For this review, take the finished solid that the model builds, in its own axes (mm). Face numbers are marked on the shaded views. A direction names the side the tool comes from. Give positions to 0.01 mm unless a question says otherwise; leave off trailing zeros. Loops run counter-clockwise (first coordinate to the right, second up) from the corner with the lowest first, then second, coordinate; pieces in that order, holes last. Notation, with made-up numbers: (-24, 78) - (1, 78) arc R8 cw to (1, 91) - close; hole circle Ø8 at (27.5, 17). An arc over 180 degrees is marked (long way). Put each result on its own line as item: value.
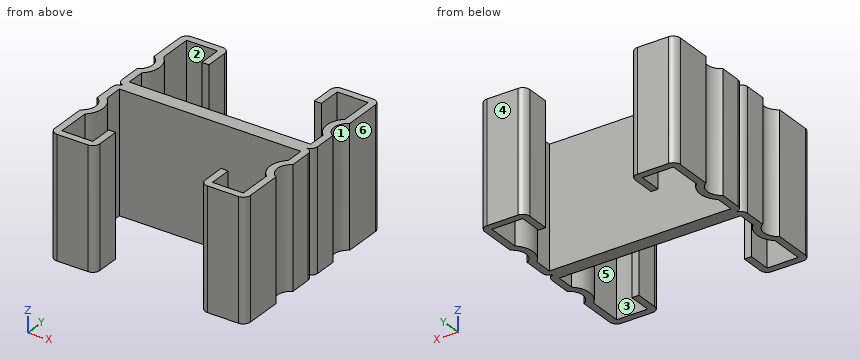
from build123d import *

# Parameters (mm, degrees)
BASE_EXTRUDE_DEPTH = 12.7


with BuildPart() as part:
    # Sketch1 → Base-Extrude (new, symmetric)
    with BuildSketch(Plane.XY):
        with BuildLine():
            Line((-20.6375, 19.1389), (-20.6375, 11.29515134))
            ThreePointArc((-20.6375, 11.29515134), (-19.1389, 8.6995), (-20.6375, 6.10384866))
            Line((-20.6375, 6.10384866), (-20.6375, 1.4986))
            ThreePointArc((-20.6375, 1.4986), (-20.198570222, 0.438929778), (-19.1389, 0))
            Line((-19.1389, 0), (19.1389, 0))
            ThreePointArc((19.1389, 0), (20.198570222, 0.438929778), (20.6375, 1.4986))
            Line((20.6375, 1.4986), (20.6375, 6.10384866))
            ThreePointArc((20.6375, 6.10384866), (19.1389, 8.6995), (20.6375, 11.29515134))
            Line((20.6375, 11.29515134), (20.6375, 19.1389))
            ThreePointArc((20.6375, 19.1389), (20.198570222, 20.198570222), (19.1389, 20.6375))
            Line((19.1389, 20.6375), (12.6111, 20.6375))
            ThreePointArc((12.6111, 20.6375), (11.551429778, 20.198570222), (11.1125, 19.1389))
            Line((11.1125, 19.1389), (11.1125, 14.2875))
            Line((11.1125, 14.2875), (12.6111, 14.2875))
            Line((12.6111, 14.2875), (12.6111, 19.1389))
            Line((12.6111, 19.1389), (19.1389, 19.1389))
            Line((19.1389, 19.1389), (19.1389, 12.050471471))
            ThreePointArc((19.1389, 12.050471471), (17.6403, 8.6995), (19.1389, 5.348528529))
            Line((19.1389, 5.348528529), (19.1389, 1.4986))
            Line((19.1389, 1.4986), (-19.1389, 1.4986))
            Line((-19.1389, 1.4986), (-19.1389, 5.348528529))
            ThreePointArc((-19.1389, 5.348528529), (-17.6403, 8.6995), (-19.1389, 12.050471471))
            Line((-19.1389, 12.050471471), (-19.1389, 19.1389))
            Line((-19.1389, 19.1389), (-12.6111, 19.1389))
            Line((-12.6111, 19.1389), (-12.6111, 14.2875))
            Line((-12.6111, 14.2875), (-11.1125, 14.2875))
            Line((-11.1125, 14.2875), (-11.1125, 19.1389))
            ThreePointArc((-11.1125, 19.1389), (-11.551429778, 20.198570222), (-12.6111, 20.6375))
            Line((-12.6111, 20.6375), (-19.1389, 20.6375))
            ThreePointArc((-19.1389, 20.6375), (-20.198570222, 20.198570222), (-20.6375, 19.1389))
        make_face()
    base_extrude = extrude(amount=BASE_EXTRUDE_DEPTH, both=True)

    # Mirror1: Base-Extrude across plane
    add(base_extrude.mirror(Plane.ZX))


solid = part.part
1) Take a section at A-A on y = 15. State the section outline as (x, z) points, and give its area (3 significant figures).
Geometry check:
outline: (-20.64, -12.7) - (-19.14, -12.7) - (-19.14, 12.7) - (-20.64, 12.7) - close; (-12.61, -12.7) - (-11.11, -12.7) - (-11.11, 12.7) - (-12.61, 12.7) - close; (11.11, -12.7) - (12.61, -12.7) - (12.61, 12.7) - (11.11, 12.7) - close; (19.14, -12.7) - (20.64, -12.7) - (20.64, 12.7) - (19.14, 12.7) - close
area: 152 mm²
2) Take a section at B-B on y = 2.5. State the section outline as (x, z) points.
Geometry check:
outline: (-20.64, -12.7) - (-19.14, -12.7) - (-19.14, 12.7) - (-20.64, 12.7) - close; (19.14, -12.7) - (20.64, -12.7) - (20.64, 12.7) - (19.14, 12.7) - close
3) Take a section at C-C on x = -5. State the section outline as (y, z) points.
Geometry check:
outline: (-1.5, -12.7) - (1.5, -12.7) - (1.5, 12.7) - (-1.5, 12.7) - close
4) Draft analysis for pull direction X (two halves, no side actions). For the marked faces 1, 2, 3 and 4, state which applies: pulls with the +X half, pulls with the -X half, needs draft (parallel to the pull), parting line crosses it, or undercut.
Geometry check:
face 1: pulls with the +X half
face 2: undercut
face 3: undercut
face 4: needs draft
5) For the marked faces 5 and 6, list the 3-axis set-ups (+Z, -Z, +X, -X, +Y, -Y) from which the entire face can be reached by the end or side of a thin tool; tool diameter is ignored.
Geometry check:
face 5: +Z, -Z
face 6: +Z, -Z, +X, +Y, -Y
6) Wall thickness on line 1 (Y direction, x = 13, z = -0.5); line 2 (X direction, y = 14.5, z = -4.5); line 3 (X direction, y = -8.5, z = -8.5): over which ranges is each line inside the solid? List them lowest first.
Geometry check:
line 1: y = -20.64 to -19.14, -1.5 to 1.5, 19.14 to 20.64
line 2: x = -20.64 to -19.14, -12.61 to -11.11, 11.11 to 12.61, 19.14 to 20.64
line 3: x = -19.15 to -17.64, 17.64 to 19.15
7) Insertion check: pin 1 Ø6 at (x, z) = (-11, 1.5) entering from +Y; pin 2 Ø12.5 at (x, z) = (0.5, -0.5) entering from -Y. Each pin has a flat end and moves straight along its axis. Give the tip position at first contact, or say it passes through.
Geometry check:
pin 1: stops at y = 20.64
pin 2: stops at y = -1.5
